Verification items for the finished model (mm, model axes). A direction names the side the tool comes from. Coordinates: 2 decimals unless noted, no trailing zeros. Order: outer loops, then holes, each group sorted by start corner. A loop starts at its lowest first (then second) coordinate and runs counter-clockwise, first axis right, second up.
Q1. Depth check by flat-ended pin: P1, Ø1, axis at x = 75.5, z = -1, coming from the -Y side; P2, Ø2.5, axis at x = -82.55, y = -19.84, coming from the +Z side; P3, Ø4, axis at x = -30.5, y = 42, coming from the +Z side (3 decimals); P4, Ø5.5, axis at x = 2.5, y = 55.5, coming from the +Z side. Enter the tip coordinate at first touch or a pass-through.
Q2. Cross-section at A-A, the plane z = 14. Record the boundary of the cut face in (x, y).
Q3. Cross-section at C-C, the plane x = 27.5. Record the boundary of the cut face in (y, z) (3 decimals), and give its area (3 significant figures).
Q4. Cross-section at B-B, the plane y = -3.5. Record the boundary of the cut face in (x, z) (1 decimal).
Q5. Draft check along X on faces 1 (the flat face through (87.312, -9, 3)), 2 (the flat face through (75, -29.369, -2)), 3 (the flat face through (-82, -29.369, 11)). Enter one of: pulls with the +X half, pulls with the -X half, needs draft (parallel to the pull), parting line crosses it, or undercut.
Q6. Set-up check for faces 4 (the flat face through (73.025, -1, -2)), 5 (the flat face through (-1, 30.956, 2)), 6 (the flat face through (2, 51, 0)): record each of +Z, -Z, +X, -X, +Y, -Y from which the full face is reachable in a straight line by a thin tool's end or side.
Q7. Thickness scan on line 1 (Y direction, x = -82.55, z = 1.75); line 2 (X direction, y = 12, z = -0.5) (1 decimal); line 3 (X direction, y = -30.5, z = 6.25). Record the ranges inside material, lowest first.
from build123d import *

# Parameters (mm, degrees)
F0_R     = 1.5875
F1_DEPTH = 3.175
F2_DEPTH = 3.175
F3_DEPTH = 19.05


# Not quite as in the source:
# - a feature names something its author has since deleted; it is built from what else it names


with BuildPart() as f1:
    # F0 (on Top) → F1 (new body)
    with BuildSketch(Plane.XY):
        Polygon((-73.025, 26.19375), (73.025, 26.19375), (73.025, -26.19375), (73.025, -29.36875), (77.7875, -29.36875), (77.7875, -26.19375), (77.7875, 30.95625), (-77.7875, 30.95625), (-77.7875, -26.19375), (-77.7875, -29.36875), (-73.025, -29.36875), (-73.025, -26.19375), align=None)
        with BuildLine():
            Line((77.7875, -26.19375), (77.7875, -29.36875))
            Line((77.7875, -29.36875), (87.3125, -29.36875))
            Line((87.3125, -29.36875), (87.3125, -26.19375))
            Line((87.3125, -26.19375), (87.3125, 34.1312500767))
            ThreePointArc((87.3125, 34.1312500767), (85.452628083, 38.621378083), (80.9625000767, 40.48125))
            Line((80.9625000767, 40.48125), (9.525, 40.48125))
            Line((9.525, 40.48125), (7.9375, 40.48125))
            Line((7.9375, 40.48125), (4.3422256552, 40.48125))
            Line((4.3422256552, 40.48125), (-1.5875, 40.48125))
            Line((-1.5875, 40.48125), (-4.3422256552, 40.48125))
            Line((-4.3422256552, 40.48125), (-9.525, 40.48125))
            Line((-9.525, 40.48125), (-80.9625000767, 40.48125))
            ThreePointArc((-80.9625000767, 40.48125), (-85.452628083, 38.621378083), (-87.3125, 34.1312500767))
            Line((-87.3125, 34.1312500767), (-87.3125, -26.19375))
            Line((-87.3125, -26.19375), (-87.3125, -29.36875))
            Line((-87.3125, -29.36875), (-77.7875, -29.36875))
            Line((-77.7875, -29.36875), (-77.7875, -26.19375))
            Line((-77.7875, -26.19375), (-77.7875, 30.95625))
            Line((-77.7875, 30.95625), (77.7875, 30.95625))
            Line((77.7875, 30.95625), (77.7875, -26.19375))
        make_face()
        with Locations((-82.55, -19.84375)):
            Circle(F0_R, mode=Mode.SUBTRACT)
        with Locations((82.55, -19.84375)):
            Circle(F0_R, mode=Mode.SUBTRACT)
        with Locations((-82.55, 34.13125)):
            Circle(F0_R, mode=Mode.SUBTRACT)
        with Locations((82.55, 34.13125)):
            Circle(F0_R, mode=Mode.SUBTRACT)
        Polygon((-77.7875, -32.54375), (-77.7875, -29.36875), (-87.3125, -29.36875), (-87.3125, -32.54375), (-87.3125, -35.71875), (-77.7875, -35.71875), align=None)
        Polygon((87.3125, -29.36875), (77.7875, -29.36875), (77.7875, -32.54375), (77.7875, -35.71875), (87.3125, -35.71875), (87.3125, -32.54375), align=None)
        Polygon((7.9375, 40.48125), (9.525, 40.48125), (0, 65.88125), (-9.525, 40.48125), (-4.3422256552, 40.48125), (0, 52.0605184138), (4.3422256552, 40.48125), align=None)
    extrude(amount=-F1_DEPTH)

    # F0 (on Top) → F2 (join)
    with BuildSketch(Plane.XY):
        with BuildLine():
            Line((77.7875, -26.19375), (77.7875, -29.36875))
            Line((77.7875, -29.36875), (87.3125, -29.36875))
            Line((87.3125, -29.36875), (87.3125, -26.19375))
            Line((87.3125, -26.19375), (87.3125, 34.1312500767))
            ThreePointArc((87.3125, 34.1312500767), (85.452628083, 38.621378083), (80.9625000767, 40.48125))
            Line((80.9625000767, 40.48125), (9.525, 40.48125))
            Line((9.525, 40.48125), (7.9375, 40.48125))
            Line((7.9375, 40.48125), (4.3422256552, 40.48125))
            Line((4.3422256552, 40.48125), (-1.5875, 40.48125))
            Line((-1.5875, 40.48125), (-4.3422256552, 40.48125))
            Line((-4.3422256552, 40.48125), (-9.525, 40.48125))
            Line((-9.525, 40.48125), (-80.9625000767, 40.48125))
            ThreePointArc((-80.9625000767, 40.48125), (-85.452628083, 38.621378083), (-87.3125, 34.1312500767))
            Line((-87.3125, 34.1312500767), (-87.3125, -26.19375))
            Line((-87.3125, -26.19375), (-87.3125, -29.36875))
            Line((-87.3125, -29.36875), (-77.7875, -29.36875))
            Line((-77.7875, -29.36875), (-77.7875, -26.19375))
            Line((-77.7875, -26.19375), (-77.7875, 30.95625))
            Line((-77.7875, 30.95625), (77.7875, 30.95625))
            Line((77.7875, 30.95625), (77.7875, -26.19375))
        make_face()
        with Locations((-82.55, -19.84375)):
            Circle(F0_R, mode=Mode.SUBTRACT)
        with Locations((82.55, -19.84375)):
            Circle(F0_R, mode=Mode.SUBTRACT)
        with Locations((-82.55, 34.13125)):
            Circle(F0_R, mode=Mode.SUBTRACT)
        with Locations((82.55, 34.13125)):
            Circle(F0_R, mode=Mode.SUBTRACT)
    extrude(amount=F2_DEPTH)

    # F0 (on Top) → F3 (join)
    with BuildSketch(Plane.XY):
        Polygon((87.3125, -29.36875), (77.7875, -29.36875), (77.7875, -32.54375), (77.7875, -35.71875), (87.3125, -35.71875), (87.3125, -32.54375), align=None)
        Polygon((-77.7875, -32.54375), (-77.7875, -29.36875), (-87.3125, -29.36875), (-87.3125, -32.54375), (-87.3125, -35.71875), (-77.7875, -35.71875), align=None)
    extrude(amount=F3_DEPTH)


solid = f1.part
Check values:
1. P1: stops at y = -29.37
1. P2: passes through
1. P3: stops at z = 3.175
1. P4: stops at z = 0
2. outline: (-87.31, -35.72) - (-77.79, -35.72) - (-77.79, -29.37) - (-87.31, -29.37) - close; (77.79, -35.72) - (87.31, -35.72) - (87.31, -29.37) - (77.79, -29.37) - close
3. outline: (26.194, -3.175) - (40.481, -3.175) - (40.481, 3.175) - (30.956, 3.175) - (30.956, 0) - (26.194, 0) - close
3. area: 75.6 mm2
4. outline: (-87.3, -3.2) - (-73, -3.2) - (-73, 0) - (-77.8, 0) - (-77.8, 3.2) - (-87.3, 3.2) - close; (73, -3.2) - (87.3, -3.2) - (87.3, 3.2) - (77.8, 3.2) - (77.8, 0) - (73, 0) - close
5. face 1: pulls with the +X half
5. face 2: undercut
5. face 3: needs draft
6. face 4: +Z, -Z, -Y
6. face 5: +Z, -Y
6. face 6: +Z, +X, -X, +Y
7. line 1: y = -35.72 to -21.43, -18.26 to 32.54, 35.72 to 40.28
7. line 2: x = -87.3 to -73, 73 to 87.3
7. line 3: x = -87.31 to -77.79, 77.79 to 87.31
